The model under review builds one solid part; all positions refer to its coordinate system, in mm. Round coordinates to 2 decimals unless told otherwise and drop trailing zeros. Write each loop counter-clockwise with the first axis right and the second up, starting at its lowest first coordinate (ties: lowest second). Pieces come first, ordered by that corner, then holes. Notation, with made-up numbers: (69, 35.25) - (95, 35.25) arc R15 cw to (95, 41.25) - close; hole circle Ø6 at (59, 85.25). An arc over 180 degrees is marked (long way). Use one line per item in the form item = value.
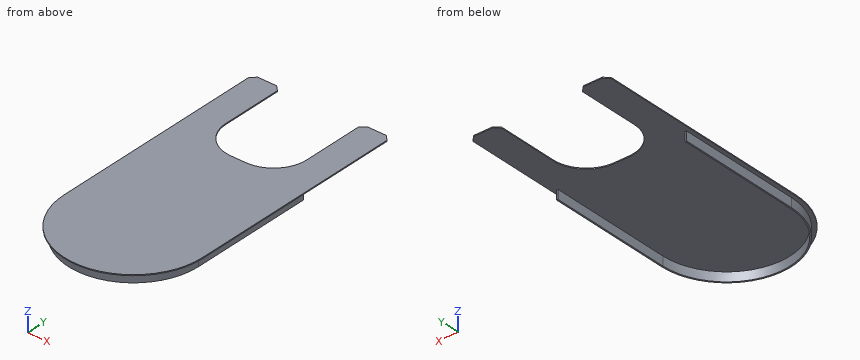
from build123d import *

# Parameters (mm, degrees)
PAD_DEPTH    = 5.5
THICKNESS_T  = -0.86
PAD001_DEPTH = 0.6
SKETCH002_W  = 17.5
SKETCH002_H  = 60
PAD002_DEPTH = 0.6
CHAMFER_SIZE = 3
FILLET_R     = 20


with BuildPart() as part:
    # Sketch → Pad (new body)
    with BuildSketch(Plane.XY):
        with BuildLine():
            Line((-39.5, 75.5), (-39.5, 0))
            ThreePointArc((-39.5, 0), (0, -39.5), (39.5, 0))
            Line((39.5, 0), (39.5, 75.5))
            Line((39.5, 75.5), (-39.5, 75.5))
        make_face()
    extrude(amount=-PAD_DEPTH)

    # Thickness
    thickness_openings = [part.faces().sort_by_distance(p)[0] for p in [
        (0, 21.873555, 0),
        (0, 75.5, -2.75),
        (0, 21.873555, -5.5),
    ]]
    offset(amount=THICKNESS_T, openings=thickness_openings)

    # Sketch001 → Pad001 (join)
    with BuildSketch(Plane.XY):
        with BuildLine():
            Line((-42, 75.5), (-42, 0))
            ThreePointArc((-42, 0), (0, -42), (42, 0))
            Line((42, 0), (42, 75.5))
            Line((42, 75.5), (-42, 75.5))
        make_face()
    extrude(amount=PAD001_DEPTH)

    # Sketch002 → Pad002 (join)
    with BuildSketch(Plane.XY):
        with Locations((-33.25, 105.5)):
            Rectangle(SKETCH002_W, SKETCH002_H)
    pad002 = extrude(amount=PAD002_DEPTH)

    # Mirrored: Pad002 across Sketch002 V_Axis
    add(pad002.mirror(Plane(origin=(0, 0, 0), x_dir=(0, 0, 1), z_dir=(1, 0, 0))))

    # Chamfer
    chamfer_edges = [part.edges().sort_by_distance(p)[0] for p in [
        (-24.5, 135.5, 0.3),
        (24.5, 135.5, 0.3),
        (-42, 135.5, 0.3),
        (42, 135.5, 0.3),
    ]]
    chamfer(chamfer_edges, length=CHAMFER_SIZE)

    # Fillet
    fillet_edges = [part.edges().sort_by_distance(p)[0] for p in [
        (24.5, 75.5, 0.3),
        (-24.5, 75.5, 0.3),
    ]]
    fillet(fillet_edges, radius=FILLET_R)


solid = part.part
(1) Add section A-A on y = 64.5. Write out the cut boundary in (x, z).
Geometry results:
outline = (-42, 0) - (-39.5, 0) - (-39.5, -5.5) - (-38.64, -5.5) - (-38.64, 0) - (38.64, 0) - (38.64, -5.5) - (39.5, -5.5) - (39.5, 0) - (42, 0) - (42, 0.6) - (-42, 0.6) - close
(2) Add section B-B on x = 0. Write out the cut boundary in (y, z).
Geometry results:
outline = (-42, 0) - (-39.5, 0) - (-39.5, -5.5) - (-38.64, -5.5) - (-38.64, 0) - (75.5, 0) - (75.5, 0.6) - (-42, 0.6) - close
(3) Add section D-D on y = 93. Write out the cut boundary in (x, z).
Geometry results:
outline = (-42, 0) - (-24.34, 0) - (-24.34, 0.6) - (-42, 0.6) - close; (24.34, 0) - (42, 0) - (42, 0.6) - (24.34, 0.6) - close
(4) Add section C-C on z = -2. Write out the cut boundary in (x, y), then the cut area to 3 significant figures.
Geometry results:
outline = (-39.5, 0) arc R39.5 ccw to (39.5, 0) - (39.5, 75.5) - (38.64, 75.5) - (38.64, 0) arc R38.64 cw to (-38.64, 0) - (-38.64, 75.5) - (-39.5, 75.5) - close
area = 235 mm2
(5) To check wall thickness, follow L1, parallel to X at y = 22, z = -4; L2, parallel to Z at x = -35, y = 3.5; L3, parallel to X at y = -33, z = -1. State the ranges of each line that lie inside material, in increasing order.
Geometry results:
L1 = -39.5 to -38.64, 38.64 to 39.5
L2 = 0 to 0.6
L3 = -21.71 to -20.1, 20.1 to 21.71
(6) Insertion check: P1, Ø1.5, axis at x = -20.5, z = -1.5, coming from the -Y side; P2, Ø0.7, axis at x = -39, z = -2, coming from the +Y side; P3, Ø25, axis at x = -17.5, y = 27.5, coming from the -Z side. Each pin has a flat end and moves straight along its axis. Give the tip position at first contact, or say it passes through.
Geometry results:
P1 = -34.21
P2 = 75.5
P3 = 0
